Drawing for the job (mm, zero at the part's lowest x, y, z). Round coordinates to 2 decimals unless told otherwise and drop trailing zeros. Loops run counter-clockwise (first coordinate to the right, second up) from the corner with the lowest first, then second, coordinate; pieces in that order, holes last. Notation, with made-up numbers: (49, 1.25) - (100, 1.25) arc R36 cw to (100, 37.25) - close; hole circle Ø4 at (-13, -34.75). An arc over 180 degrees is marked (long way). Put each result on its own line as item: value.
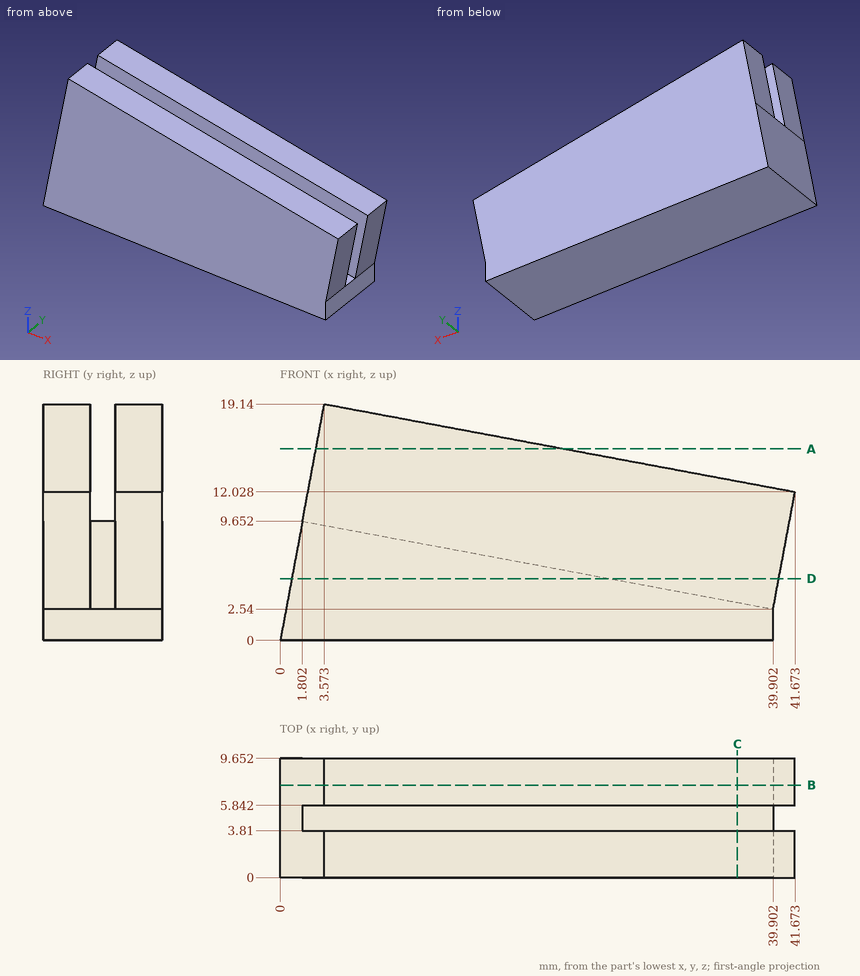
1. Band-saw the part on B-B (y = 7.5). List the corners of the cut face in (x, z), plus the area to 3 significant figures.
A:
outline: (0, 0) - (39.9, 0) - (39.9, 2.54) - (41.67, 12.03) - (3.57, 19.14) - close
area: 615 mm²
2. Pin check, flat tips, straight feed: P1, Ø1, axis at x = 37, y = 8, coming from the +Z side; P2, Ø2, axis at y = 4.5, z = 8, coming from the -X side; P3, Ø4, axis at x = 33.5, y = 6.5, coming from the +Z side. Stop position of each tip, or through.
A:
P1: stops at z = 12.99
P2: stops at x = 1.31
P3: stops at z = 13.93
3. Band-saw the part on A-A (z = 15.5). List the corners of the cut face in (x, y).
A:
outline: (2.89, 0) - (23.07, 0) - (23.07, 3.81) - (2.89, 3.81) - close; (2.89, 5.84) - (23.07, 5.84) - (23.07, 9.65) - (2.89, 9.65) - close
4. Probe line 1 along Y through (x, z) = (7.5, 17); line 2 along Z through (x, y) = (39, 4); line 3 along Z through (x, y) = (30, 3.25). List the from-to ranges inside material, lowest first. Write a range as [from, to].
A:
line 1: y = [0, 3.81], [5.84, 9.65]
line 2: z = [0, 2.71]
line 3: z = [0, 14.21]
5. Band-saw the part on C-C (x = 37). List the corners of the cut face in (y, z), plus the area to 3 significant figures.
A:
outline: (0, 0) - (9.65, 0) - (9.65, 12.9) - (5.84, 12.9) - (5.84, 3.08) - (3.81, 3.08) - (3.81, 12.9) - (0, 12.9) - close
area: 105 mm²
6. Band-saw the part on D-D (z = 5). List the corners of the cut face in (x, y), plus the area to 3 significant figures.
A:
outline: (0.93, 0) - (40.36, 0) - (40.36, 3.81) - (26.72, 3.81) - (26.72, 5.84) - (40.36, 5.84) - (40.36, 9.65) - (0.93, 9.65) - close
area: 353 mm²
